```python
from build123d import *
from OCP.BRepFilletAPI import BRepFilletAPI_MakeChamfer

# Parameters (mm, degrees)
Z_KLAD_PROTA_EN_DEPTH    = 10
SKICA2_R                 = 1.875
ODEBR_N_PROTA_EN_1_DEPTH = 1.1
ODEBR_N_PROTA_EN_2_DEPTH = 0.5
SKICA4_W                 = 2.1
SKICA4_H                 = 3
SKICA4_W_2               = 1.2
SKICA4_H_2               = 1
ODEBR_N_PROTA_EN_3_DEPTH = 0.5
SKICA5_W                 = 2.8
SKICA5_H                 = 2
ODEBR_N_PROTA_EN_4_DEPTH = 1
LINE_RN_POLE1_COUNT      = 3
LINE_RN_POLE1_PITCH      = 5
ZKOSEN_1_SIZE            = 1.2
ZKOSEN_1_SIZE_2          = 1
ZKOSEN_2_SIZE            = 0.5
ZKOSEN_2_SIZE_2          = 1
SKICA6_W                 = 2.1
SKICA6_H                 = 1.3
ODEBR_N_PROTA_EN_5_DEPTH = 2
LINE_RN_POLE2_COUNT      = 3
LINE_RN_POLE2_PITCH      = 5
SKICA7_W                 = 0.6
SKICA7_H                 = 1
P_ID_N_PROTA_EN_1_DEPTH  = 4.8
LINE_RN_POLE3_COUNT      = 2
LINE_RN_POLE3_PITCH      = 5
ZKOSEN_3_SIZE            = 0.2
ZKOSEN_3_SIZE2           = 0.115470054


# Some blends are built 0.0001 mm under size
with BuildPart() as part:
    # Skica1 → Základ-Protažení (new body)
    with BuildSketch(Plane.XY):
        Polygon((-2.5, 10), (2.5, 10), (3.3, 5.3), (4, 5.3), (4, 0), (-4, 0), (-4, 5.3), (-3, 5.3), (-3, 7.3), align=None)
    extrude(amount=Z_KLAD_PROTA_EN_DEPTH)

    # Skica2 → Odebrání-Protažení1 (cut)
    with BuildSketch(Plane(origin=(0, 10, 0), x_dir=(-1, 0, 0), z_dir=(0, 1, 0))):
        with Locations(Location((0, 2.5, 0), (0, 0, 90))):
            Circle(SKICA2_R)
        with Locations(Location((0, 7.5, 0), (0, 0, 90))):
            Circle(SKICA2_R)
    extrude(amount=-ODEBR_N_PROTA_EN_1_DEPTH, mode=Mode.SUBTRACT)

    # Skica3 → Odebrání-Protažení2 (cut)
    with BuildSketch(Plane(origin=(0, 8.9, 0), x_dir=(-1, 0, 0), z_dir=(0, 1, 0))):
        Polygon((1.814998003, 2.029460683), (-1.314998003, 3.83656472), (-1.814998003, 2.970539317), (1.314998003, 1.16343528), align=None)
        Polygon((-1.314998003, 8.83656472), (1.814998003, 7.029460683), (1.314998003, 6.16343528), (-1.814998003, 7.970539317), align=None)
    extrude(amount=-ODEBR_N_PROTA_EN_2_DEPTH, mode=Mode.SUBTRACT)

    # Skica4 → Odebrání-Protažení3 (cut)
    with BuildSketch(Plane.ZY.offset(4)):
        with Locations((7.5, 3.8)):
            Rectangle(SKICA4_W, SKICA4_H)
        with Locations((7.5, 0.5)):
            Rectangle(SKICA4_W_2, SKICA4_H_2)
        with Locations((2.5, 3.8)):
            Rectangle(SKICA4_W, SKICA4_H)
        with Locations((2.5, 0.5)):
            Rectangle(SKICA4_W_2, SKICA4_H_2)
        with Locations((-2.5, 3.8)):
            Rectangle(SKICA4_W, SKICA4_H)
        with Locations((-2.5, 0.5)):
            Rectangle(SKICA4_W_2, SKICA4_H_2)
    extrude(amount=-ODEBR_N_PROTA_EN_3_DEPTH, mode=Mode.SUBTRACT)

    # Skica5 → Odebrání-Protažení4 (cut)
    with BuildSketch(Plane(origin=(4, 0, 0), x_dir=(0, 0, -1), z_dir=(1, 0, 0))):
        with Locations((-7.5, 2.5)):
            Rectangle(SKICA5_W, SKICA5_H)
    odebr_n_prota_en_4 = extrude(amount=-ODEBR_N_PROTA_EN_4_DEPTH, mode=Mode.SUBTRACT)

    # Lineární Pole1: Odebrání-Protažení4 ×3
    with Locations(*[(0, 0, -i * LINE_RN_POLE1_PITCH) for i in range(1, LINE_RN_POLE1_COUNT)]):
        add(odebr_n_prota_en_4, mode=Mode.SUBTRACT)

    # Zkosení1
    # the kernel refuses this chamfer: 1.2, 1 mm, written as the material it adds along each edge
    # the kernel refuses this chamfer: 1.2, 1 mm, written as the material it takes off along each edge
    with BuildSketch(Plane(origin=(4, 3.5, 8.9), x_dir=(0.024836286378920516, 0.9996915318631564, 0), z_dir=(0, 0, -1)), Plane(origin=(4, 3.5, 3.9), x_dir=(0.024836286378920516, 0.9996915318631564, 0), z_dir=(0, 0, -1))) as zkosen_1_2_piece_1:
        Polygon((ZKOSEN_1_SIZE * 0.999691531863, -ZKOSEN_1_SIZE * 0.0248362863789), (-ZKOSEN_1_SIZE_2 * 0.0248362863789, -ZKOSEN_1_SIZE_2 * 0.999691531863), (0, 0), align=None)
    extrude(amount=2.8, mode=Mode.SUBTRACT)
    with BuildSketch(Plane(origin=(4, 3.5, 11.993140689), x_dir=(0.024836286378920505, 0.9996915318631564, 0), z_dir=(0, 0, -1))) as zkosen_1_2_piece_2_section:
        Polygon((ZKOSEN_1_SIZE * 0.999691531863, -ZKOSEN_1_SIZE * 0.0248362863789), (-ZKOSEN_1_SIZE_2 * 0.0248362863789, -ZKOSEN_1_SIZE_2 * 0.999691531863), (0, 0), align=None)
    zkosen_1_2_piece_2 = extrude(amount=8.986281378, mode=Mode.PRIVATE)
    zkosen_1_2_piece_2 = split(zkosen_1_2_piece_2, bisect_by=Plane(origin=(3.666666667, 3.9, 3.9), z_dir=(0, 0, -1)), keep=Keep.TOP, mode=Mode.PRIVATE)
    add(zkosen_1_2_piece_2, mode=Mode.SUBTRACT)
    with BuildSketch(Plane(origin=(4, 3.5, 6.993140689), x_dir=(0.024836286378920505, 0.9996915318631564, 0), z_dir=(0, 0, -1))) as zkosen_1_2_piece_3_section:
        Polygon((ZKOSEN_1_SIZE * 0.999691531863, -ZKOSEN_1_SIZE * 0.0248362863789), (-ZKOSEN_1_SIZE_2 * 0.0248362863789, -ZKOSEN_1_SIZE_2 * 0.999691531863), (0, 0), align=None)
    zkosen_1_2_piece_3 = extrude(amount=8.986281378, mode=Mode.PRIVATE)
    zkosen_1_2_piece_3 = split(zkosen_1_2_piece_3, bisect_by=Plane(origin=(3.666666667, 3.9, 6.1), z_dir=(0, 0, 1)), keep=Keep.TOP, mode=Mode.PRIVATE)
    add(zkosen_1_2_piece_3, mode=Mode.SUBTRACT)

    # Zkosení2
    zkosen_2_edges_1 = [part.edges().sort_by_distance(p)[0] for p in [
        (4, 3.1, 8.9),
    ]]
    zkosen_2_side_1 = [part.faces().sort_by_distance(p)[0] for p in [
        (4, 3.1, 8.91),
    ]]
    zkosen_2_edges_2 = [part.edges().sort_by_distance(p)[0] for p in [
        (4, 1.5, 7.5),
    ]]
    zkosen_2_side_2 = [part.faces().sort_by_distance(p)[0] for p in [
        (4, 1.49, 7.5),
    ]]
    zkosen_2_edges_3 = [part.edges().sort_by_distance(p)[0] for p in [
        (4, 3.1, 6.1),
    ]]
    zkosen_2_side_3 = [part.faces().sort_by_distance(p)[0] for p in [
        (4, 3.1, 6.09),
    ]]
    zkosen_2_edges_4 = [part.edges().sort_by_distance(p)[0] for p in [
        (4, 3.1, 3.9),
    ]]
    zkosen_2_side_4 = [part.faces().sort_by_distance(p)[0] for p in [
        (4, 3.1, 3.91),
    ]]
    zkosen_2_edges_5 = [part.edges().sort_by_distance(p)[0] for p in [
        (4, 1.5, 2.5),
    ]]
    zkosen_2_side_5 = [part.faces().sort_by_distance(p)[0] for p in [
        (4, 1.49, 2.5),
    ]]
    zkosen_2_edges_6 = [part.edges().sort_by_distance(p)[0] for p in [
        (4, 3.1, 1.1),
    ]]
    zkosen_2_side_6 = [part.faces().sort_by_distance(p)[0] for p in [
        (4, 3.1, 1.09),
    ]]
    zkosen_2 = BRepFilletAPI_MakeChamfer(part.part.solid().wrapped)
    for e in zkosen_2_edges_1:
        zkosen_2.Add(ZKOSEN_2_SIZE - 0.0001, ZKOSEN_2_SIZE_2 - 0.0001, e.wrapped, zkosen_2_side_1[0].wrapped)
    for e in zkosen_2_edges_2:
        zkosen_2.Add(ZKOSEN_2_SIZE - 0.0001, ZKOSEN_2_SIZE_2 - 0.0001, e.wrapped, zkosen_2_side_2[0].wrapped)
    for e in zkosen_2_edges_3:
        zkosen_2.Add(ZKOSEN_2_SIZE - 0.0001, ZKOSEN_2_SIZE_2 - 0.0001, e.wrapped, zkosen_2_side_3[0].wrapped)
    for e in zkosen_2_edges_4:
        zkosen_2.Add(ZKOSEN_2_SIZE - 0.0001, ZKOSEN_2_SIZE_2 - 0.0001, e.wrapped, zkosen_2_side_4[0].wrapped)
    for e in zkosen_2_edges_5:
        zkosen_2.Add(ZKOSEN_2_SIZE - 0.0001, ZKOSEN_2_SIZE_2 - 0.0001, e.wrapped, zkosen_2_side_5[0].wrapped)
    for e in zkosen_2_edges_6:
        zkosen_2.Add(ZKOSEN_2_SIZE - 0.0001, ZKOSEN_2_SIZE_2 - 0.0001, e.wrapped, zkosen_2_side_6[0].wrapped)
    add(Compound.cast(zkosen_2.Shape()), mode=Mode.REPLACE)  # a hair under: the kernel refuses the full size

    # Skica6 → Odebrání-Protažení5 (cut)
    with BuildSketch(Plane(origin=(3, 0, 0), x_dir=(0, 0, -1), z_dir=(1, 0, 0))):
        with Locations((-7.45, 2.55)):
            Rectangle(SKICA6_W, SKICA6_H)
    odebr_n_prota_en_5 = extrude(amount=-ODEBR_N_PROTA_EN_5_DEPTH, mode=Mode.SUBTRACT)

    # Lineární Pole2: Odebrání-Protažení5 ×3
    with Locations(*[(0, 0, -i * LINE_RN_POLE2_PITCH) for i in range(1, LINE_RN_POLE2_COUNT)]):
        add(odebr_n_prota_en_5, mode=Mode.SUBTRACT)

    # Skica7 → Přidání-Protažení1 (add)
    with BuildSketch(Plane.XZ):
        with Locations((0, 2.5)):
            Rectangle(SKICA7_W, SKICA7_H)
    p_id_n_prota_en_1 = extrude(amount=P_ID_N_PROTA_EN_1_DEPTH)

    # Lineární Pole3: Přidání-Protažení1 ×2
    with Locations(*[(0, 0, i * LINE_RN_POLE3_PITCH) for i in range(1, LINE_RN_POLE3_COUNT)]):
        add(p_id_n_prota_en_1)

    # Zkosení3: one chamfer whose edges measure the first distance from different faces: ONE call of the kernel's chamfer builder (chamfer() names one face for all edges)
    zkosen_3_edges_1 = [part.edges().sort_by_distance(p)[0] for p in [
        (0, -4.8, 2),
    ]]
    zkosen_3_side_1 = [part.faces().sort_by_distance(p)[0] for p in [
        (0, -2.4, 2),
    ]]
    zkosen_3_edges_2 = [part.edges().sort_by_distance(p)[0] for p in [
        (0, -4.8, 3),
    ]]
    zkosen_3_side_2 = [part.faces().sort_by_distance(p)[0] for p in [
        (0, -2.4, 3),
    ]]
    zkosen_3_edges_3 = [part.edges().sort_by_distance(p)[0] for p in [
        (0, -4.8, 7),
    ]]
    zkosen_3_side_3 = [part.faces().sort_by_distance(p)[0] for p in [
        (0, -2.4, 7),
    ]]
    zkosen_3_edges_4 = [part.edges().sort_by_distance(p)[0] for p in [
        (0, -4.8, 8),
    ]]
    zkosen_3_side_4 = [part.faces().sort_by_distance(p)[0] for p in [
        (0, -2.4, 8),
    ]]
    zkosen_3 = BRepFilletAPI_MakeChamfer(part.part.solid().wrapped)
    for e in zkosen_3_edges_1:
        zkosen_3.Add(ZKOSEN_3_SIZE, ZKOSEN_3_SIZE2, e.wrapped, zkosen_3_side_1[0].wrapped)  # the first distance lies on this face
    for e in zkosen_3_edges_2:
        zkosen_3.Add(ZKOSEN_3_SIZE, ZKOSEN_3_SIZE2, e.wrapped, zkosen_3_side_2[0].wrapped)  # the first distance lies on this face
    for e in zkosen_3_edges_3:
        zkosen_3.Add(ZKOSEN_3_SIZE, ZKOSEN_3_SIZE2, e.wrapped, zkosen_3_side_3[0].wrapped)  # the first distance lies on this face
    for e in zkosen_3_edges_4:
        zkosen_3.Add(ZKOSEN_3_SIZE, ZKOSEN_3_SIZE2, e.wrapped, zkosen_3_side_4[0].wrapped)  # the first distance lies on this face
    add(Compound.cast(zkosen_3.Shape()), mode=Mode.REPLACE)


solid = part.part
```
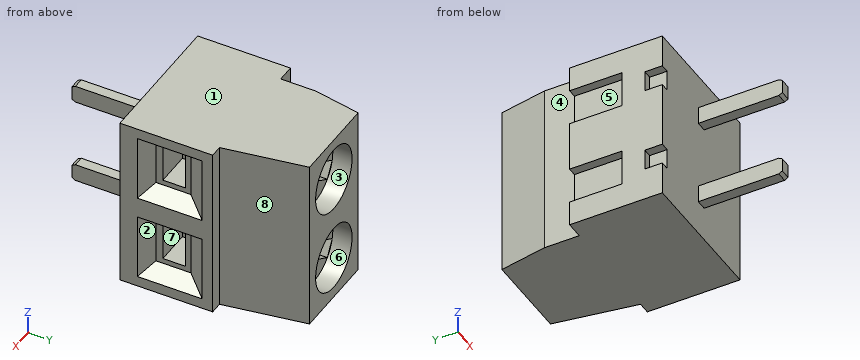
Input: part model. Units: mm. Frame: model coordinates. Face numbers are marked on the shaded views. A direction names the side the tool comes from. Coordinates: 2 decimals unless noted, no trailing zeros. Order: outer loops, then holes, each group sorted by start corner. A loop starts at its lowest first (then second) coordinate and runs counter-clockwise, first axis right, second up. Notation, with made-up numbers: (37, -6) - (47, -6) arc R20 ccw to (47, 22) - close; hole circle Ø5 at (-19.5, 82.25). An arc over 180 degrees is marked (long way). Put each result on its own line as item: value.
1. Reachability of the marked faces 5, 6, 7 and 8 from +Z, -Z, +X, -X, +Y, -Y: full face, straight path, thin tool, end or side. Return the list, or none.
Report:
face 5: -X, +Y
face 6: +Y
face 7: +X
face 8: +Z, -Z, +X, +Y
2. Draft query along X for the marked faces 1, 2, 3 and 4. Return one class per face: pulls with the +X half, pulls with the -X half, needs draft (parallel to the pull), parting line crosses it, or undercut.
Report:
face 1: needs draft
face 2: pulls with the +X half
face 3: undercut
face 4: pulls with the -X half
3. Line query: line 1 along Z through (x, y) = (0, 9.55) (3 decimals); line 2 along Y through (x, z) = (2.25, 7.5); line 3 along X through (y, z) = (6.5, 2.75). Output: solid intervals per line, ascending.
Report:
line 1: z = 0 to 0.625, 4.375 to 5.625, 9.375 to 10
line 2: y = 0 to 1.9, 3.2 to 10
line 3: x = -3 to 3.1
4. Cut plane B-B on x = 3.5. Return the cut outline in (y, z), then the cut area to 3 significant figures.
Report:
outline: (0, 0) - (5.3, 0) - (5.3, 10) - (0, 10) - close; hole (1.25, 0.85) - (4.1, 0.85) - (4.1, 4.15) - (1.25, 4.15) - close; hole (1.25, 5.85) - (4.1, 5.85) - (4.1, 9.15) - (1.25, 9.15) - close
area: 34.2 mm2
5. Contact query for flat-ended pins moving along their axis: pin 1 Ø2 at (x, z) = (-0.5, 7) entering from +Y; pin 2 Ø4 at (x, z) = (2.5, 1.5) entering from -Y; pin 3 Ø3 at (x, z) = (0, 3) entering from +Y; pin 4 Ø1.6 at (y, z) = (2.5, 8) entering from +X. Output: stop coordinate, or through.
Report:
pin 1: stops at y = 8.9
pin 2: stops at y = 0
pin 3: stops at y = 10
pin 4: stops at x = 3
6. Cut plane D-D on x = 1.5. Return the cut outline in (y, z) (3 decimals).
Report:
outline: (0, 0) - (10, 0) - (10, 1.375) - (8.9, 1.375) - (8.9, 2.789) - (8.4, 2.789) - (8.4, 3.516) - (8.9, 3.516) - (8.9, 3.625) - (10, 3.625) - (10, 6.375) - (8.9, 6.375) - (8.9, 7.789) - (8.4, 7.789) - (8.4, 8.516) - (8.9, 8.516) - (8.9, 8.625) - (10, 8.625) - (10, 10) - (0, 10) - close; hole (1.9, 1.4) - (3.2, 1.4) - (3.2, 3.5) - (1.9, 3.5) - close; hole (1.9, 6.4) - (3.2, 6.4) - (3.2, 8.5) - (1.9, 8.5) - close
